Design review of the part built by this model. Coordinates are the model's own, in mm. A direction names the side the tool comes from. Round coordinates to 2 decimals unless told otherwise and drop trailing zeros. Order: outer loops, then holes, each group sorted by start corner. A loop starts at its lowest first (then second) coordinate and runs counter-clockwise, first axis right, second up.
from build123d import *

# Parameters (mm, degrees)
SKETCH1_R           = 2.35
BOSS_EXTRUDE1_DEPTH = 19.4
SKETCH2_R           = 4
BOSS_EXTRUDE2_DEPTH = 2
CHAMFER1_SIZE       = 0.5
SKETCH3_R           = 1.5
CUT_EXTRUDE1_DEPTH  = 4


with BuildPart() as part:
    # Sketch1 → Boss-Extrude1 (new body)
    with BuildSketch(Plane(origin=(0, 0, 0), x_dir=(1, 0, 0), z_dir=(0, 1, 0))):
        with Locations(Location((0, 0, 0), (0, 0, 270))):
            Circle(SKETCH1_R)
    extrude(amount=BOSS_EXTRUDE1_DEPTH)

    # Sketch2 → Boss-Extrude2 (add)
    with BuildSketch(Plane(origin=(0, 19.4, 0), x_dir=(1, 0, 0), z_dir=(0, 1, 0))):
        with Locations(Location((0, 0, 0), (0, 0, 270))):
            Circle(SKETCH2_R)
    extrude(amount=BOSS_EXTRUDE2_DEPTH)

    # Chamfer1
    chamfer1_edges = [part.edges().sort_by_distance(p)[0] for p in [
        (0, 21.4, -4),
    ]]
    chamfer(chamfer1_edges, length=CHAMFER1_SIZE)

    # Sketch3 → Cut-Extrude1 (cut)
    with BuildSketch(Plane.XZ):
        with Locations(Location((0, 0, 0), (0, 0, 270))):
            Circle(SKETCH3_R)
    extrude(amount=-CUT_EXTRUDE1_DEPTH, mode=Mode.SUBTRACT)


solid = part.part
1) To check wall thickness, follow line 1 along X through (y, z) = (1.95, 0); line 2 along Y through (x, z) = (-2, -1.5); line 3 along X through (y, z) = (1.5, 1). State the ranges of each line that lie inside material, in increasing order.
Results:
line 1: x = -2.35 to -1.5, 1.5 to 2.35
line 2: y = 19.4 to 21.4
line 3: x = -2.13 to -1.12, 1.12 to 2.13
2) Take a section at C-C on x = 0. Give the boundary of the cut face in (y, z).
Results:
outline: (0, -2.35) - (19.4, -2.35) - (19.4, -4) - (20.9, -4) - (21.4, -3.5) - (21.4, 3.5) - (20.9, 4) - (19.4, 4) - (19.4, 2.35) - (0, 2.35) - (0, 1.5) - (4, 1.5) - (4, -1.5) - (0, -1.5) - close
3) Take a section at D-D on y = 9. Give the boundary of the cut face in (x, z), plus the area to 3 significant figures.
Results:
outline: circle Ø4.7 at (0, 0)
area: 17.3 mm2
4) Take a section at B-B on y = 3. Give the boundary of the cut face in (x, z).
Results:
outline: circle Ø4.7 at (0, 0); hole circle Ø3 at (0, 0)
5) The part is to be moulded in two halves that separate along Z. For faces 3 (the face through (-3.905, 20.14, -0.867)), 4 (the face through (-2, 0, 0)), 5 (the face through (0.45, 1.97, -1.43)), 6 (the face through (0, 4, 0)), say which applies: released by +Z, released by -Z, zero draft, split by the parting line, or undercut.
Results:
face 3: split by the parting line
face 4: zero draft
face 5: undercut
face 6: undercut
6) For faces 1 (the face through (-2, 19.4, 2)), 2 (the face through (0, 21.4, 0)), list the 3-axis set-ups (+Z, -Z, +X, -X, +Y, -Y) from which the entire face can be reached by the end or side of a thin tool; tool diameter is ignored.
Results:
face 1: -Y
face 2: +Z, -Z, +X, -X, +Y
7) Clearance check with flat-ended pins moving along their axes: P1, Ø2.5, axis at x = 0, z = 0, coming from the -Y side; P2, Ø1, axis at x = -0.5, y = 12, coming from the +Z side. State where each tip first meets the part, or that it passes through.
Results:
P1: stops at y = 4
P2: stops at z = 2.35
8) Take a section at A-A on z = 0. Give the boundary of the cut face in (x, y).
Results:
outline: (-4, 19.4) - (-2.35, 19.4) - (-2.35, 0) - (-1.5, 0) - (-1.5, 4) - (1.5, 4) - (1.5, 0) - (2.35, 0) - (2.35, 19.4) - (4, 19.4) - (4, 20.9) - (3.5, 21.4) - (-3.5, 21.4) - (-4, 20.9) - close
